Build history of the part. All positions in model axes, mm. Give positions to 0.01 mm unless a question says otherwise; leave off trailing zeros. Write each loop counter-clockwise with the first axis right and the second up, starting at its lowest first coordinate (ties: lowest second). Pieces come first, ordered by that corner, then holes. Notation, with made-up numbers: (8, 39.25) -> (67, 39.25) arc R18 ccw to (67, 43.25) -> close; hole circle Ø9 at (29, 6). An arc over 180 degrees is marked (long way). Put each result on its own line as item: value.
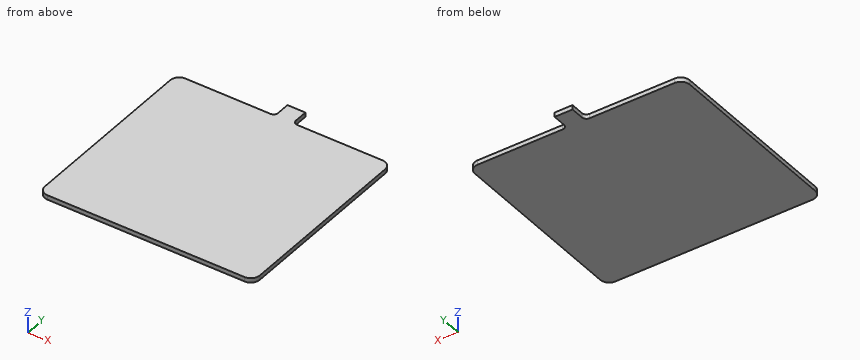
from build123d import *

# Parameters (mm, degrees)
BOSS_EXTRU_1_DEPTH = 10


with BuildPart() as part:
    # Esquisse1 → Boss.-Extru.1 (new body)
    with BuildSketch(Plane.XY):
        with BuildLine():
            Line((-220, 295), (-30, 295))
            ThreePointArc((-30, 295), (-22.928932188, 297.928932188), (-20, 305))
            Line((-20, 305), (-20, 335))
            Line((-20, 335), (20, 335))
            Line((20, 335), (20, 305))
            ThreePointArc((20, 305), (22.928932188, 297.928932188), (30, 295))
            Line((30, 295), (220, 295))
            ThreePointArc((220, 295), (234.142135624, 289.142135624), (240, 275))
            Line((240, 275), (240, -125))
            ThreePointArc((240, -125), (234.142135624, -139.142135624), (220, -145))
            Line((220, -145), (-220, -145))
            ThreePointArc((-220, -145), (-234.142135624, -139.142135624), (-240, -125))
            Line((-240, -125), (-240, 275))
            ThreePointArc((-240, 275), (-234.142135624, 289.142135624), (-220, 295))
        make_face()
    extrude(amount=BOSS_EXTRU_1_DEPTH)


solid = part.part
1) Slice it at B-B (x = 86). Write the cut outline in (y, z), plus the area to 3 significant figures.
Filled sheet:
outline: (-145, 0) -> (295, 0) -> (295, 10) -> (-145, 10) -> close
area: 4,400 mm2
2) Wall check: L1, parallel to Y at x = 74.5, z = 0.5. Give the ranges that are in metal, low to high.
Filled sheet:
L1: -145 to 295
3) Pin check, flat tips, straight feed: pin 1 (1.5 mm diameter, centred on x = 52.5, z = 1.5, fed in from +Y); pin 2 (3 mm diameter, centred on y = 318, z = 5.5, fed in from -X); pin 3 (10 mm diameter, centred on x = 32.5, y = 13, fed in from -Z); pin 4 (3 mm diameter, centred on y = 312.5, z = 5, fed in from +X). Stop position of each tip, or through.
Filled sheet:
pin 1: y = 295
pin 2: x = -20
pin 3: z = 0
pin 4: x = 20
4) Slice it at A-A (z = 6). Write the cut outline in (x, y).
Filled sheet:
outline: (-240, -125) arc R20 ccw to (-220, -145) -> (220, -145) arc R20 ccw to (240, -125) -> (240, 275) arc R20 ccw to (220, 295) -> (30, 295) arc R10 cw to (20, 305) -> (20, 335) -> (-20, 335) -> (-20, 305) arc R10 cw to (-30, 295) -> (-220, 295) arc R20 ccw to (-240, 275) -> close
